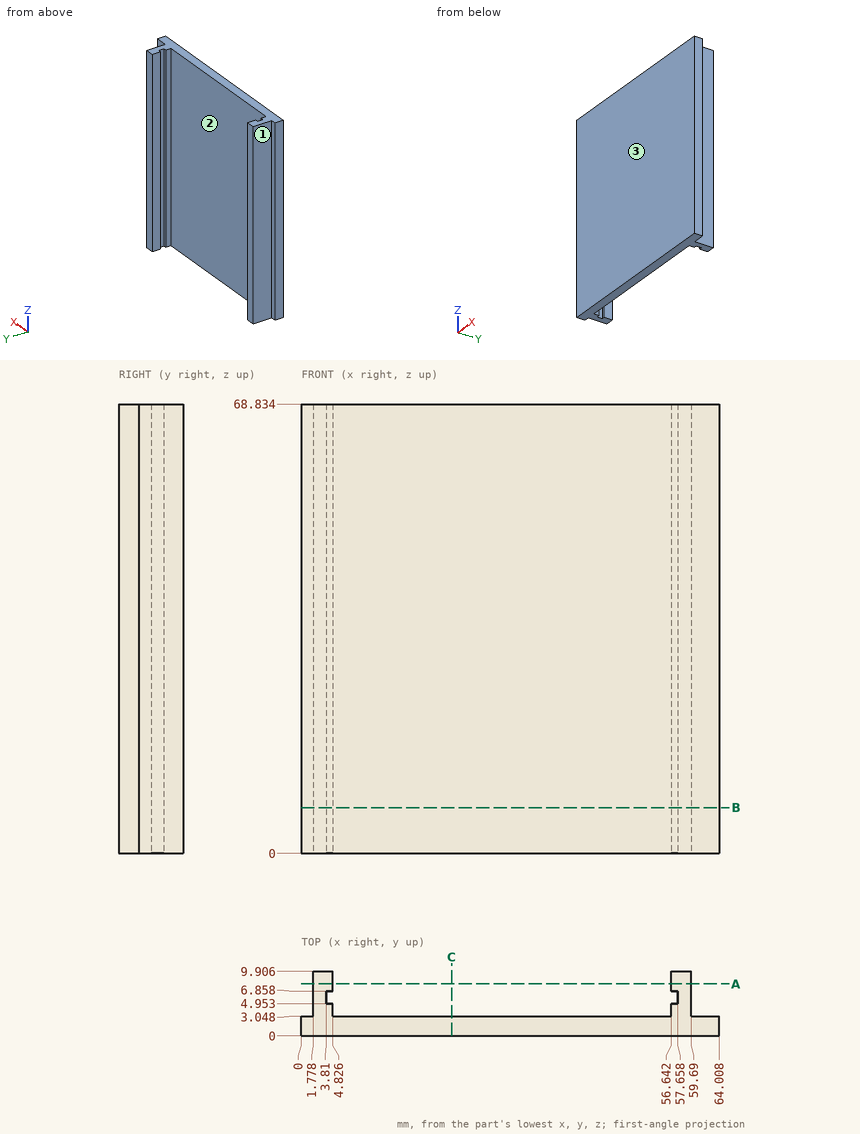
Geometry check sheet. Reference: drawing and pictorial views, mm from the part's lowest x, y, z. Give positions to 0.01 mm unless a question says otherwise; leave off trailing zeros. Order: outer loops, then holes, each group sorted by start corner. A loop starts at its lowest first (then second) coordinate and runs counter-clockwise, first axis right, second up. Notation, with made-up numbers: M -19.75,43 L 0.25,43 A22 cw 0.25,74 Z; hole C 75,-13.5 d6. An arc over 180 degrees is marked long. Answer in a Markdown table with one row per item. Add a question column.
Item 1: Gauge pin test, flat ends, axial feed: pin 1 (1 mm diameter, centred on x = 10, z = 56, fed in from +Y); pin 2 (2.5 mm diameter, centred on y = 8.5, z = 21, fed in from +X); pin 3 (2.5 mm diameter, centred on y = 8, z = 26.5, fed in from -X). Record the tip position at first contact, or that the pin passes through.
Item 2: Scan lines: probe 1 along X at (y, z) = (7.75, 58); probe 2 along X at (y, z) = (5.25, 7); probe 3 along Y at (x, z) = (49, 37). Record each from-to range of solid material in increasing order. Write a range as from..to.
Item 3: Section check A-A, the plane y = 8. Enter the section's corners in (x, z), and give its area (3 significant figures).
Item 4: Section check C-C, the plane x = 23. Enter the section's corners in (y, z), and give its area (3 significant figures).
Item 5: Mould release check, pull along X, two halves, no side actions. Record for the marked faces 1, 2 and 3: released by +X, released by -X, zero draft, split by the parting line, or undercut.
Item 6: Section check B-B, the plane z = 7. Enter the section's corners in (x, y), and give its area (3 significant figures).
Filled sheet:
| question | item | result |
|---|---|---|
| 1 | pin 1 | stops at y = 3.05 |
| 1 | pin 2 | stops at x = 59.69 |
| 1 | pin 3 | stops at x = 1.78 |
| 2 | probe 1 | x = 1.78..4.83, 56.64..59.69 |
| 2 | probe 2 | x = 1.78..3.81, 57.66..59.69 |
| 2 | probe 3 | y = 0..3.05 |
| 3 | outline | M 1.78,0 L 4.83,0 L 4.83,68.83 L 1.78,68.83 Z; M 56.64,0 L 59.69,0 L 59.69,68.83 L 56.64,68.83 Z |
| 3 | area | 420 mm^2 |
| 4 | outline | M 0,0 L 3.05,0 L 3.05,68.83 L 0,68.83 Z |
| 4 | area | 210 mm^2 |
| 5 | face 1 | released by -X |
| 5 | face 2 | undercut |
| 5 | face 3 | zero draft |
| 6 | outline | M 0,0 L 64.01,0 L 64.01,3.05 L 59.69,3.05 L 59.69,9.91 L 56.64,9.91 L 56.64,6.86 L 57.66,6.86 L 57.66,4.95 L 56.64,4.95 L 56.64,3.05 L 4.83,3.05 L 4.83,4.95 L 3.81,4.95 L 3.81,6.86 L 4.83,6.86 L 4.83,9.91 L 1.78,9.91 L 1.78,3.05 L 0,3.05 Z |
| 6 | area | 233 mm^2 |
